from build123d import *

# Parameters (mm, degrees)
F0_R     = 11.2
F1_DEPTH = 7


with BuildPart() as f1:
    # F0 (on Top) → F1 (new body)
    with BuildSketch(Plane.XY):
        with BuildLine():
            ThreePointArc((-10.5879527755, -12.2611278447), (-14.0296115413, -8.1), (-15.9124245803, -3.0388721553))
            ThreePointArc((-15.9124245803, -3.0388721553), (-24.9741529622, 0.8279459046), (-34.6003773558, -1.2703884587))
            ThreePointArc((-34.6003773558, -1.2703884587), (-40.5299888971, -23.4), (-18.4003773558, -29.3296115413))
            ThreePointArc((-18.4003773558, -29.3296115413), (-12.4707658145, -23.4), (-10.3003773558, -15.3))
            ThreePointArc((-10.3003773558, -15.3), (-10.3724314512, -13.7737756064), (-10.5879527755, -12.2611278447))
        make_face()
        with Locations((-26.5003773558, -15.3)):
            Circle(F0_R, mode=Mode.SUBTRACT)
        with BuildLine():
            ThreePointArc((-15.9124245803, -3.0388721553), (-16.1279459046, -1.5262243936), (-16.2, 0))
            Line((-16.2, 0), (-16.2, 9.3530743609))
            Line((-16.2, 9.3530743609), (-34.6003773558, -1.2703884587))
            ThreePointArc((-34.6003773558, -1.2703884587), (-24.9741529622, 0.8279459046), (-15.9124245803, -3.0388721553))
        make_face()
        with BuildLine():
            ThreePointArc((-10.5879527755, -12.2611278447), (-12.4707658145, -7.2), (-15.9124245803, -3.0388721553))
            ThreePointArc((-15.9124245803, -3.0388721553), (-14.0296115413, -8.1), (-10.5879527755, -12.2611278447))
        make_face()
        with BuildLine():
            ThreePointArc((5.3244718048, 15.3), (2.7, 14.6265845856), (0, 14.4))
            ThreePointArc((0, 14.4), (-2.7, 14.6265845856), (-5.3244718048, 15.3))
            ThreePointArc((-5.3244718048, 15.3), (-6.7422238556, 14.730323061), (-8.1, 14.0296115413))
            ThreePointArc((-8.1, 14.0296115413), (-14.0296115413, 8.1), (-16.2, 0))
            ThreePointArc((-16.2, 0), (-16.1279459046, -1.5262243936), (-15.9124245803, -3.0388721553))
            ThreePointArc((-15.9124245803, -3.0388721553), (-12.4707658145, -7.2), (-10.5879527755, -12.2611278447))
            ThreePointArc((-10.5879527755, -12.2611278447), (-9.385722049, -13.2040986674), (-8.1, -14.0296115413))
            ThreePointArc((-8.1, -14.0296115413), (0, -16.2), (8.1, -14.0296115413))
            ThreePointArc((8.1, -14.0296115413), (9.385722049, -13.2040986674), (10.5879527755, -12.2611278447))
            ThreePointArc((10.5879527755, -12.2611278447), (12.4707658145, -7.2), (15.9124245803, -3.0388721553))
            ThreePointArc((15.9124245803, -3.0388721553), (16.1279459046, -1.5262243936), (16.2, 0))
            ThreePointArc((16.2, 0), (14.0296115413, 8.1), (8.1, 14.0296115413))
            ThreePointArc((8.1, 14.0296115413), (6.7422238556, 14.730323061), (5.3244718048, 15.3))
        make_face()
        with BuildLine():
            ThreePointArc((0, 11.2), (7.9195959493, 7.9195959493), (11.2, 0))
            ThreePointArc((11.2, 0), (-7.9195959493, -7.9195959493), (0, 11.2))
        make_face(mode=Mode.SUBTRACT)
        with BuildLine():
            ThreePointArc((-16.2, 0), (-14.0296115413, 8.1), (-8.1, 14.0296115413))
            Line((-8.1, 14.0296115413), (-16.2, 9.3530743609))
            Line((-16.2, 9.3530743609), (-16.2, 0))
        make_face()
        with BuildLine():
            ThreePointArc((-8.1, 14.0296115413), (-6.7422238556, 14.730323061), (-5.3244718048, 15.3))
            ThreePointArc((-5.3244718048, 15.3), (-13.2040986674, 21.214277951), (-16.2, 30.6))
            Line((-16.2, 30.6), (-16.2, 9.3530743609))
            Line((-16.2, 9.3530743609), (-8.1, 14.0296115413))
        make_face()
        with BuildLine():
            Line((0, 16.2), (0, 14.4))
            ThreePointArc((0, 14.4), (2.7, 14.6265845856), (5.3244718048, 15.3))
            ThreePointArc((5.3244718048, 15.3), (2.7, 15.9734154144), (0, 16.2))
        make_face()
        with BuildLine():
            ThreePointArc((-5.3244718048, 15.3), (-2.7, 14.6265845856), (0, 14.4))
            Line((0, 14.4), (0, 16.2))
            ThreePointArc((0, 16.2), (-2.7, 15.9734154144), (-5.3244718048, 15.3))
        make_face()
        with BuildLine():
            ThreePointArc((-5.3244718048, 15.3), (-2.7, 15.9734154144), (0, 16.2))
            Line((0, 16.2), (0, 19.4))
            ThreePointArc((0, 19.4), (-11.2, 30.6), (0, 41.8))
            Line((0, 41.8), (0, 46.8))
            ThreePointArc((0, 46.8), (-11.4551298552, 42.0551298552), (-16.2, 30.6))
            ThreePointArc((-16.2, 30.6), (-13.2040986674, 21.214277951), (-5.3244718048, 15.3))
        make_face()
        with BuildLine():
            Line((0, 19.4), (0, 16.2))
            ThreePointArc((0, 16.2), (2.7, 15.9734154144), (5.3244718048, 15.3))
            ThreePointArc((5.3244718048, 15.3), (13.2040986674, 21.214277951), (16.2, 30.6))
            ThreePointArc((16.2, 30.6), (11.4551298552, 42.0551298552), (0, 46.8))
            Line((0, 46.8), (0, 41.8))
            ThreePointArc((0, 41.8), (7.9195959493, 38.5195959493), (11.2, 30.6))
            ThreePointArc((11.2, 30.6), (7.9195959493, 22.6804040507), (0, 19.4))
        make_face()
        with BuildLine():
            Line((16.2, 9.3530743609), (8.1, 14.0296115413))
            ThreePointArc((8.1, 14.0296115413), (14.0296115413, 8.1), (16.2, 0))
            Line((16.2, 0), (16.2, 9.3530743609))
        make_face()
        with BuildLine():
            ThreePointArc((16.2, 30.6), (13.2040986674, 21.214277951), (5.3244718048, 15.3))
            ThreePointArc((5.3244718048, 15.3), (6.7422238556, 14.730323061), (8.1, 14.0296115413))
            Line((8.1, 14.0296115413), (16.2, 9.3530743609))
            Line((16.2, 9.3530743609), (16.2, 30.6))
        make_face()
        with BuildLine():
            Line((16.2, 9.3530743609), (16.2, 0))
            ThreePointArc((16.2, 0), (16.1279459046, -1.5262243936), (15.9124245803, -3.0388721553))
            ThreePointArc((15.9124245803, -3.0388721553), (24.9741529622, 0.8279459046), (34.6003773558, -1.2703884587))
            Line((34.6003773558, -1.2703884587), (16.2, 9.3530743609))
        make_face()
        with BuildLine():
            ThreePointArc((18.4003773558, -29.3296115413), (11.7700542948, -22.0422238556), (10.5879527755, -12.2611278447))
            ThreePointArc((10.5879527755, -12.2611278447), (9.385722049, -13.2040986674), (8.1, -14.0296115413))
            Line((8.1, -14.0296115413), (0, -18.7061487217))
            Line((0, -18.7061487217), (18.4003773558, -29.3296115413))
        make_face()
        with BuildLine():
            ThreePointArc((-8.1, -14.0296115413), (-9.385722049, -13.2040986674), (-10.5879527755, -12.2611278447))
            ThreePointArc((-10.5879527755, -12.2611278447), (-10.3724314512, -13.7737756064), (-10.3003773558, -15.3))
            ThreePointArc((-10.3003773558, -15.3), (-12.4707658145, -23.4), (-18.4003773558, -29.3296115413))
            Line((-18.4003773558, -29.3296115413), (0, -18.7061487217))
            Line((0, -18.7061487217), (-8.1, -14.0296115413))
        make_face()
        with BuildLine():
            ThreePointArc((34.6003773558, -1.2703884587), (24.9741529622, 0.8279459046), (15.9124245803, -3.0388721553))
            ThreePointArc((15.9124245803, -3.0388721553), (14.0296115413, -8.1), (10.5879527755, -12.2611278447))
            ThreePointArc((10.5879527755, -12.2611278447), (11.7700542948, -22.0422238556), (18.4003773558, -29.3296115413))
            ThreePointArc((18.4003773558, -29.3296115413), (34.6003773558, -29.3296115413), (42.7003773558, -15.3))
            ThreePointArc((42.7003773558, -15.3), (40.5299888971, -7.2), (34.6003773558, -1.2703884587))
        make_face()
        with Locations((26.5003773558, -15.3)):
            Circle(F0_R, mode=Mode.SUBTRACT)
        with BuildLine():
            ThreePointArc((8.1, -14.0296115413), (0, -16.2), (-8.1, -14.0296115413))
            Line((-8.1, -14.0296115413), (0, -18.7061487217))
            Line((0, -18.7061487217), (8.1, -14.0296115413))
        make_face()
        with BuildLine():
            ThreePointArc((10.5879527755, -12.2611278447), (14.0296115413, -8.1), (15.9124245803, -3.0388721553))
            ThreePointArc((15.9124245803, -3.0388721553), (12.4707658145, -7.2), (10.5879527755, -12.2611278447))
        make_face()
    extrude(amount=F1_DEPTH)


solid = f1.part
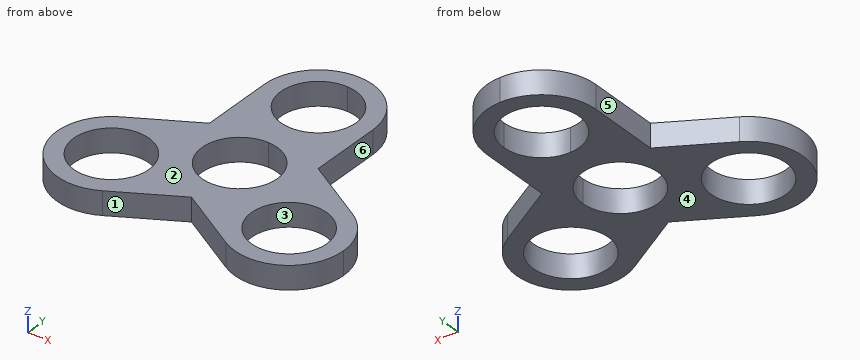
The model under review builds one solid part; all positions refer to its coordinate system, in mm. Face numbers are marked on the shaded views. A direction names the side the tool comes from. Round coordinates to 2 decimals unless told otherwise and drop trailing zeros. Order: outer loops, then holes, each group sorted by start corner. A loop starts at its lowest first (then second) coordinate and runs counter-clockwise, first axis right, second up. Notation, with made-up numbers: (48.5, 24.25) - (70.5, 24.25) arc R21 cw to (70.5, 49.25) - close; hole circle Ø8 at (10, 23). An arc over 180 degrees is marked (long way). Use one line per item in the form item = value.
Q1. Add section C-C on x = 8.5. Give the boundary of the cut face in (y, z).
Response values:
outline = (-23.61, 0) - (-7.29, 0) - (-7.29, 7) - (-23.61, 7) - close; (7.29, 0) - (23.31, 0) - (23.31, 7) - (7.29, 7) - close; (37.89, 0) - (44.39, 0) - (44.39, 7) - (37.89, 7) - close
Q2. Add section B-B on z = 5. Give the boundary of the cut face in (x, y), then the cut area to 3 significant figures.
Response values:
outline = (-34.6, -1.27) arc R16.2 ccw to (-18.4, -29.33) - (0, -18.71) - (18.4, -29.33) arc R16.2 ccw to (34.6, -1.27) - (16.2, 9.35) - (16.2, 30.6) arc R16.2 ccw to (-16.2, 30.6) - (-16.2, 9.35) - close; hole circle Ø22.4 at (-26.5, -15.3); hole circle Ø22.4 at (0, 0); hole circle Ø22.4 at (0, 30.6); hole circle Ø22.4 at (26.5, -15.3)
area = 2,180 mm^2
Q3. Add section A-A on y = 25. Give the boundary of the cut face in (x, z).
Response values:
outline = (-16.2, 0) - (-9.7, 0) - (-9.7, 7) - (-16.2, 7) - close; (9.7, 0) - (16.2, 0) - (16.2, 7) - (9.7, 7) - close
Q4. Tool access review of the marked faces 1 and 2: name each direction out of +Z, -Z, +X, -X, +Y, -Y from which nothing blocks a thin tool from reaching the whole face with its end or side.
Response values:
face_1 = +Z, -Z, -Y
face_2 = +Z, +X, -X, +Y, -Y
Q5. Mouldability with a two-part tool opening along X and no side actions: class the marked faces 3, 4, 5 and 6 as pulls with the +X half, pulls with the -X half, needs draft (parallel to the pull), parting line crosses it, or undercut.
Response values:
face_3 = undercut
face_4 = needs draft
face_5 = pulls with the -X half
face_6 = pulls with the +X half
Q6. Clearance check with flat-ended pins moving along their axes: P1, Ø1.5, axis at y = 4.5, z = 4.5, coming from the +X side; P2, Ø2, axis at y = -18.5, z = 3.5, coming from the -X side. State where each tip first meets the part, or that it passes through.
Response values:
P1 = 25.9
P2 = -42.55
Q7. Add section D-D on x = 26. Give the boundary of the cut face in (y, z).
Response values:
outline = (-31.49, 0) - (-26.49, 0) - (-26.49, 7) - (-31.49, 7) - close; (-4.11, 0) - (3.7, 0) - (3.7, 7) - (-4.11, 7) - close
Q8. To check wall thickness, follow line 1 (Y direction, x = 2, z = 2.75); line 2 (X direction, y = -13.5, z = 4.75); line 3 (X direction, y = -5.5, z = 1.75). State the ranges of each line that lie inside material, in increasing order.
Response values:
line_1 = -19.86 to -11.02, 11.02 to 19.58, 41.62 to 46.68
line_2 = -42.6 to -37.55, -15.45 to 15.45, 37.55 to 42.6
line_3 = -39.4 to -31.92, -21.08 to -9.76, 9.76 to 21.08, 31.92 to 39.4
